```python
from build123d import *

# Parameters (mm, degrees)
SKETCH1_R           = 25
SKETCH1_R_2         = 20
BOSS_EXTRUDE1_DEPTH = 181
SKETCH5_W           = 2.5
SKETCH5_H           = 30
CUT_EXTRUDE2_DEPTH  = 6
CIRPATTERN8_COUNT   = 2
CIRPATTERN8_ANGLE   = 90


with BuildPart() as part:
    # Sketch1 → Boss-Extrude1 (new body)
    with BuildSketch(Plane.XY):
        Circle(SKETCH1_R)
        Circle(SKETCH1_R_2, mode=Mode.SUBTRACT)
    extrude(amount=BOSS_EXTRUDE1_DEPTH)

    # Sketch5 → Cut-Extrude2 (cut)
    with BuildSketch(Plane(origin=(0, 22.5, 0), x_dir=(-1, 0, 0), z_dir=(0, 1, 0))):
        with Locations((0, 166.230203819)):
            Rectangle(SKETCH5_W, SKETCH5_H)
    cut_extrude2 = extrude(amount=-CUT_EXTRUDE2_DEPTH, mode=Mode.SUBTRACT)

    # CirPattern8: Cut-Extrude2 ×2 about axis
    cirpattern8_axis = Axis((0, 0, 0), (0, 0, -1))
    for i in range(1, CIRPATTERN8_COUNT):
        add(cut_extrude2.rotate(cirpattern8_axis, i * CIRPATTERN8_ANGLE / (CIRPATTERN8_COUNT - 1)), mode=Mode.SUBTRACT)


solid = part.part
```
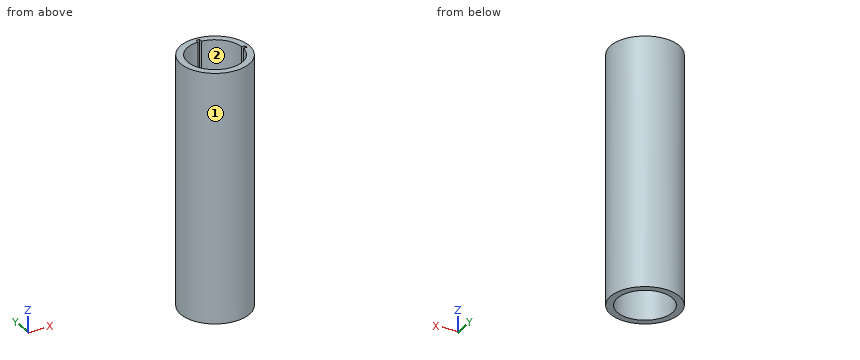
Design review of the part built by this model. Coordinates are the model's own, in mm. Face numbers are marked on the shaded views. Give positions to 0.01 mm unless a question says otherwise; leave off trailing zeros. Order: outer loops, then holes, each group sorted by start corner. A loop starts at its lowest first (then second) coordinate and runs counter-clockwise, first axis right, second up. Notation, with made-up numbers: (-2, 22) -> (48, 22) arc R12 cw to (48, 39) -> close; hole circle Ø5 at (17, -5). An arc over 180 degrees is marked (long way). Write item = value, one per line. Start each with the question number.
(1) For pin 1 (3 mm diameter, centred on x = 21.5, z = 165.5, fed in from +Y); pin 2 (1.3 mm diameter, centred on y = 21.5, z = 164, fed in from -X); pin 3 (0.8 mm diameter, centred on x = 20.5, z = 166.5, fed in from -Y); pin 4 (4 mm diameter, centred on x = -16.5, y = -2.5, fed in from +Z), all flat-tipped, find the tip position at first contact; note any pin that passes through.
(2) We need section B-B on x = 9. Write out the cut boundary in (y, z).
(3) To check wall thickness, follow line 1 along Y through (x, z) = (0, 90.5); line 2 along Y through (x, z) = (16.5, 44); line 3 along X through (y, z) = (-12, 39.5). State the ranges of each line that lie inside material, in increasing order.
(4) We need section A-A on z = 162.5. Write out the cut boundary in (x, y), plus the area to 3 significant figures.
(5) Mouldability with a two-part tool opening along Y and no side actions: class the marked faces 1 and 2 as +Y half, -Y half, draft (parallel to the pull), parting line (faces both ways), or undercut.
(6) We need section C-C on y = 12.5. Write out the cut boundary in (x, z), plus the area to 3 significant figures.
(7) We need section D-D on z = 70.5. Write out the cut boundary in (x, y), plus the area to 3 significant figures.
Numbers:
q1.pin_1 = 15
q1.pin_2 = -13.79
q1.pin_3 = -14.87
q1.pin_4 = through
q2.outline = (-23.32, 0) -> (-17.86, 0) -> (-17.86, 181) -> (-23.32, 181) -> close; (17.86, 0) -> (23.32, 0) -> (23.32, 181) -> (17.86, 181) -> close
q3.line_1 = -25 to -20, 20 to 25
q3.line_2 = -18.78 to -11.3, 11.3 to 18.78
q3.line_3 = -21.93 to -16, 16 to 21.93
q4.outline = circle Ø50 at (0, 0); hole (-1.25, 19.96) arc R20 ccw (long way) to (19.96, -1.25) -> (22.5, -1.25) -> (22.5, 1.25) -> (19.96, 1.25) arc R20 ccw to (1.25, 19.96) -> (1.25, 22.5) -> (-1.25, 22.5) -> close
q4.area = 694 mm^2
q5.face_1 = parting line
q5.face_2 = undercut
q6.outline = (-21.65, 0) -> (-15.61, 0) -> (-15.61, 181) -> (-21.65, 181) -> close; (15.61, 0) -> (21.65, 0) -> (21.65, 181) -> (15.61, 181) -> close
q6.area = 2,190 mm^2
q7.outline = circle Ø50 at (0, 0); hole circle Ø40 at (0, 0)
q7.area = 707 mm^2
